Geometry check sheet. Reference: the model listing, model coordinates, mm. A direction names the side the tool comes from. Coordinates: 2 decimals unless noted, no trailing zeros. Order: outer loops, then holes, each group sorted by start corner. A loop starts at its lowest first (then second) coordinate and runs counter-clockwise, first axis right, second up. Notation, with made-up numbers: (-22, 52.25) - (27, 52.25) arc R36 ccw to (27, 90.25) - close; hole circle Ø3 at (-37.75, -37.5). An arc over 180 degrees is marked (long way). Put each result on its own line as item: value.
from build123d import *

# Parameters (mm, degrees)
METAL_HORN_FLANGE_PROFILE_R              = 16
METAL_HORN_FLANGE_DEPTH                  = 4
STRAIGHT_FOREARM_WEB_PROFILE_W           = 28
STRAIGHT_FOREARM_WEB_PROFILE_H           = 14
STRAIGHT_FOREARM_WEB_DEPTH               = 4
REPLACEABLE_TOOL_MOUNTING_DECK_PROFILE_W = 39
REPLACEABLE_TOOL_MOUNTING_DECK_PROFILE_H = 30
REPLACEABLE_TOOL_MOUNTING_DECK_DEPTH     = 4
DOWEL_SUPPORT_HUB_START                  = 4
DOWEL_SUPPORT_HUB_PROFILE_R              = 7
DOWEL_SUPPORT_HUB_PROFILE_R_2            = 4
DOWEL_SUPPORT_HUB_DEPTH                  = 4
WASHER_SEATS_CLEAR_DOWEL_SLEEVE_START    = 4
RAISED_WASHER_SEATS_PCD14_R              = 3.5
WASHER_SEATS_CLEAR_DOWEL_SLEEVE_DEPTH    = 4
METAL_HORN_M3_PATTERN_START              = -50
METAL_HORN_M3_PATTERN_PROFILE_R          = 1.6
METAL_HORN_M3_PATTERN_DEPTH              = 115.52906322
ELBOW_SLEEVE_BORE_START                  = -50
ELBOW_SLEEVE_BORE_PROFILE_R              = 4
ELBOW_SLEEVE_BORE_DEPTH                  = 115.52906322
MODULAR_TOOL_FOUR_M3_PATTERN_START       = -50
MODULAR_TOOL_FOUR_M3_PATTERN_PROFILE_R   = 1.7
MODULAR_TOOL_FOUR_M3_PATTERN_DEPTH       = 115.52906322


with BuildPart() as part:
    # Metal_horn_flange_profile → Metal_horn_flange (new body)
    with BuildSketch(Plane.XY):
        Circle(METAL_HORN_FLANGE_PROFILE_R)
    extrude(amount=METAL_HORN_FLANGE_DEPTH)

    # Straight_forearm_web_profile → Straight_forearm_web (add)
    with BuildSketch(Plane.XY):
        with Locations((14, 0)):
            Rectangle(STRAIGHT_FOREARM_WEB_PROFILE_W, STRAIGHT_FOREARM_WEB_PROFILE_H)
    extrude(amount=STRAIGHT_FOREARM_WEB_DEPTH)

    # Replaceable_tool_mounting_deck_profile → Replaceable_tool_mounting_deck (add)
    with BuildSketch(Plane.XY):
        with Locations((42.5, 0)):
            Rectangle(REPLACEABLE_TOOL_MOUNTING_DECK_PROFILE_W, REPLACEABLE_TOOL_MOUNTING_DECK_PROFILE_H)
    extrude(amount=REPLACEABLE_TOOL_MOUNTING_DECK_DEPTH)

    # Dowel_support_hub_profile → Dowel_support_hub (add)
    with BuildSketch(Plane.XY.offset(DOWEL_SUPPORT_HUB_START)):
        Circle(DOWEL_SUPPORT_HUB_PROFILE_R)
        Circle(DOWEL_SUPPORT_HUB_PROFILE_R_2, mode=Mode.SUBTRACT)
    extrude(amount=DOWEL_SUPPORT_HUB_DEPTH)

    # Raised_washer_seats_PCD14 → Washer_seats_clear_dowel_sleeve (add)
    with BuildSketch(Plane.XY.offset(WASHER_SEATS_CLEAR_DOWEL_SLEEVE_START)):
        with Locations((7, 0)):
            Circle(RAISED_WASHER_SEATS_PCD14_R)
        with Locations((-7, 0)):
            Circle(RAISED_WASHER_SEATS_PCD14_R)
        with Locations((0, 7)):
            Circle(RAISED_WASHER_SEATS_PCD14_R)
        with Locations((0, -7)):
            Circle(RAISED_WASHER_SEATS_PCD14_R)
    extrude(amount=WASHER_SEATS_CLEAR_DOWEL_SLEEVE_DEPTH)

    # Metal_horn_M3_pattern_profile → Metal_horn_M3_pattern (cut, through all)
    with BuildSketch(Plane.XY.offset(METAL_HORN_M3_PATTERN_START)):
        with Locations(Location((7, 0, 0), (0, 0, 180))):
            Circle(METAL_HORN_M3_PATTERN_PROFILE_R)
        with Locations(Location((-7, 0, 0), (0, 0, 180))):
            Circle(METAL_HORN_M3_PATTERN_PROFILE_R)
        with Locations(Location((0, 7, 0), (0, 0, 180))):
            Circle(METAL_HORN_M3_PATTERN_PROFILE_R)
        with Locations(Location((0, -7, 0), (0, 0, 180))):
            Circle(METAL_HORN_M3_PATTERN_PROFILE_R)
    extrude(amount=METAL_HORN_M3_PATTERN_DEPTH, mode=Mode.SUBTRACT)

    # Elbow_sleeve_bore_profile → Elbow_sleeve_bore (cut, through all)
    with BuildSketch(Plane.XY.offset(ELBOW_SLEEVE_BORE_START)):
        Circle(ELBOW_SLEEVE_BORE_PROFILE_R)
    extrude(amount=ELBOW_SLEEVE_BORE_DEPTH, mode=Mode.SUBTRACT)

    # Modular_tool_four_M3_pattern_profile → Modular_tool_four_M3_pattern (cut, through all)
    with BuildSketch(Plane.XY.offset(MODULAR_TOOL_FOUR_M3_PATTERN_START)):
        with Locations(Location((27, -11.5, 0), (0, 0, 180))):
            Circle(MODULAR_TOOL_FOUR_M3_PATTERN_PROFILE_R)
        with Locations(Location((27, 11.5, 0), (0, 0, 180))):
            Circle(MODULAR_TOOL_FOUR_M3_PATTERN_PROFILE_R)
        with Locations(Location((58, -11.5, 0), (0, 0, 180))):
            Circle(MODULAR_TOOL_FOUR_M3_PATTERN_PROFILE_R)
        with Locations(Location((58, 11.5, 0), (0, 0, 180))):
            Circle(MODULAR_TOOL_FOUR_M3_PATTERN_PROFILE_R)
    extrude(amount=MODULAR_TOOL_FOUR_M3_PATTERN_DEPTH, mode=Mode.SUBTRACT)


solid = part.part
Q1. Section check C-C on z = 3.25. State how many separate pieces and enclosed holes the cut face has, then the cut area to 3 significant figures.
Answer block:
separate pieces: 1
enclosed holes: 9
area: 1,960 mm^2
Q2. Draft check along Y on faces 6 (the cylindrical face through (0.35, 8.56, 3.94)), 7 (the cylindrical face through (-0.1, -10.5, 6)), 8 (the flat face through (19, 7, 2)), 9 (the flat face through (5, 0, 8)). Enter one of: pulls with the +Y half, pulls with the -Y half, needs draft (parallel to the pull), parting line crosses it, or undercut.
Answer block:
face 6: undercut
face 7: undercut
face 8: pulls with the +Y half
face 9: needs draft
Q3. Section check D-D on x = 7. Record the boundary of the cut face in (y, z).
Answer block:
outline: (-14.39, 0) - (-1.6, 0) - (-1.6, 8) - (-3.5, 8) - (-3.5, 4) - (-14.39, 4) - close; (1.6, 0) - (14.39, 0) - (14.39, 4) - (3.5, 4) - (3.5, 8) - (1.6, 8) - close
Q4. Section check A-A on x = 58. Record the boundary of the cut face in (y, z).
Answer block:
outline: (-15, 0) - (-13.2, 0) - (-13.2, 4) - (-15, 4) - close; (-9.8, 0) - (9.8, 0) - (9.8, 4) - (-9.8, 4) - close; (13.2, 0) - (15, 0) - (15, 4) - (13.2, 4) - close
Q5. Access from +Z, -Z, +X, -X, +Y, -Y to the whole of each face (thin tool, end or side, straight path). Record for faces 1 (the flat face through (42, 15, 2)), 2 (the flat face through (62, 0, 2)), 3 (the flat face through (23, -11, 2)), 4 (the cylindrical face through (0.1, 10.5, 6)), 5 (the cylindrical face through (8.6, -0.07, 3.94)).
Answer block:
face 1: +Z, -Z, +X, +Y
face 2: +Z, -Z, +X, +Y, -Y
face 3: +Z, -Z, -Y
face 4: +Z
face 5: +Z, -Z
Q6. Section check B-B on y = -11.5. Record the boundary of the cut face in (x, z).
Answer block:
outline: (-11.12, 0) - (11.12, 0) - (11.12, 4) - (-11.12, 4) - close; (23, 0) - (25.3, 0) - (25.3, 4) - (23, 4) - close; (28.7, 0) - (56.3, 0) - (56.3, 4) - (28.7, 4) - close; (59.7, 0) - (62, 0) - (62, 4) - (59.7, 4) - close
Q7. Depth check by flat-ended pin: pin 1 Ø1.2 at (x, z) = (18, 1.5) entering from +Y; pin 2 Ø4.5 at (x, z) = (39.5, 2) entering from -Y; pin 3 Ø3 at (y, z) = (3, 5) entering from -X. Enter the tip coordinate at first touch or a pass-through.
Answer block:
pin 1: stops at y = 7
pin 2: stops at y = -15
pin 3: stops at x = -15.89
Q8. Thickness scan on L1, parallel to Y at x = 27, z = 2; L2, parallel to Y at x = 0, z = 5.25; L3, parallel to X at y = -13, z = 3.75. Record the ranges inside material, lowest first. Write a range as [from, to].
Answer block:
L1: y = [-15, -13.2], [-9.8, 9.8], [13.2, 15]
L2: y = [-10.5, -8.6], [-5.4, -4], [4, 5.4], [8.6, 10.5]
L3: x = [-9.33, 9.33], [23, 26.2], [27.8, 57.2], [58.8, 62]
